CAD build for the part. Positions are in the model's coordinates, mm. A direction names the side the tool comes from. Give positions to 0.01 mm unless a question says otherwise; leave off trailing zeros. Order: outer loops, then holes, each group sorted by start corner. A loop starts at its lowest first (then second) coordinate and runs counter-clockwise, first axis right, second up.
```python
from build123d import *

# Parameters (mm, degrees)
ESQUISSE1_W             = 49
ESQUISSE1_H             = 79
BOSS_EXTRU_1_DEPTH      = 273
ESQUISSE2_W             = 6
ESQUISSE2_H             = 273
ENL_V_MAT_EXTRU_1_DEPTH = 5


with BuildPart() as part:
    # Esquisse1 → Boss.-Extru.1 (new body)
    with BuildSketch(Plane.XY):
        with Locations((24.5, 39.5)):
            Rectangle(ESQUISSE1_W, ESQUISSE1_H)
    extrude(amount=BOSS_EXTRU_1_DEPTH)

    # Esquisse2 → Enlèv. mat.-Extru.1 (cut)
    with BuildSketch(Plane.XZ):
        with Locations((9, 136.5)):
            Rectangle(ESQUISSE2_W, ESQUISSE2_H)
        with Locations((27, 136.5)):
            Rectangle(ESQUISSE2_W, ESQUISSE2_H)
    enl_v_mat_extru_1 = extrude(amount=-ENL_V_MAT_EXTRU_1_DEPTH, mode=Mode.SUBTRACT)

    # Symétrie2: Enlèv. mat.-Extru.1 across plane
    add(enl_v_mat_extru_1.mirror(Plane(origin=(0, 39.5, 0), x_dir=(0, 0, 1), z_dir=(0, -1, 0))), mode=Mode.SUBTRACT)


solid = part.part
```
Item 1: Slice it at A-A (z = 23.5). Give the cut face in (x, y).
Item 2: Two-plate mould, pull along X, no slides. Class faces 4 (the face through (0, 39, 135)), 5 (the face through (24, 40, 273)), 6 (the face through (24, 2, 135)): released by +X, released by -X, zero draft, split by the parting line, or undercut.
Item 3: Drop flat-ended pins along their axis: pin 1 Ø1.8 at (x, z) = (25.5, 155.5) entering from +Y; pin 2 Ø4 at (x, z) = (6, 78) entering from -Y; pin 3 Ø1.8 at (x, z) = (9.5, 201.5) entering from -Y. Give the stop position or say it passes through.
Item 4: Tool access for faces 1 (the face through (39, 0, 135)), 2 (the face through (27, 74, 138)), 3 (the face through (30, 2, 135)): list every direction of +Z, -Z, +X, -X, +Y, -Y with a clear straight run to the whole face (end or side of a thin tool).
Item 5: Wall check: L1, parallel to Y at x = 26, z = 253.5. Give the ranges that are in metal, low to high.
Item 6: Slice it at B-B (x = 27). Give the cut face in (y, z).
A:
1. outline: (0, 0) - (6, 0) - (6, 5) - (12, 5) - (12, 0) - (24, 0) - (24, 5) - (30, 5) - (30, 0) - (49, 0) - (49, 79) - (30, 79) - (30, 74) - (24, 74) - (24, 79) - (12, 79) - (12, 74) - (6, 74) - (6, 79) - (0, 79) - close
2. face 4: released by -X
2. face 5: zero draft
2. face 6: undercut
3. pin 1: stops at y = 74
3. pin 2: stops at y = 0
3. pin 3: stops at y = 5
4. face 1: +Z, -Z, +X, -X, -Y
4. face 2: +Z, -Z, +Y
4. face 3: +Z, -Z, -Y
5. L1: y = 5 to 74
6. outline: (5, 0) - (74, 0) - (74, 273) - (5, 273) - close
